Design review of the part built by this model. Coordinates are the model's own, in mm. Face numbers are marked on the shaded views. A direction names the side the tool comes from. Give positions to 0.01 mm unless a question says otherwise; leave off trailing zeros. Loops run counter-clockwise (first coordinate to the right, second up) from the corner with the lowest first, then second, coordinate; pieces in that order, holes last. Notation, with made-up numbers: (62, 44.25) - (110, 44.25) arc R17 cw to (110, 71.25) - close; hole circle Ø4 at (38.25, 65.25). An arc over 180 degrees is marked (long way). Write each question's results on one line, items separated by ' | '.
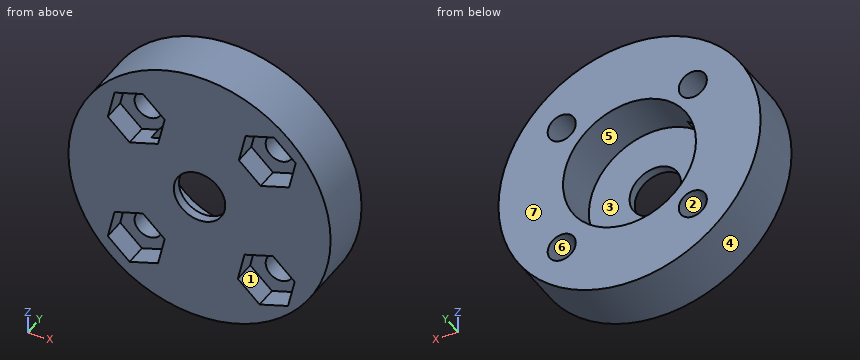
Autodesk Inventor part; units mm, degrees
ref_plane "YZ Plane" through (0, 0, 0) normal (1, 0, 0) x (0, 1, 0)
ref_plane "XZ Plane" through (0, 0, 0) normal (0, 1, 0) x (-1, 0, 0)
ref_plane "XY Plane" through (0, 0, 0) normal (0, 0, 1) x (1, 0, 0)
sketch "Эскиз1" plane through (0, 0, 0) normal (0, 1, 0) x (-1, 0, 0)
  circle A0 centre (0, 0) radius 14
  circle A1 centre (0, 0) radius 7.1
  circle A2 centre (6.7581, 6.7661) radius 1.5
  circle A3 centre (-7.2419, -7.2339) radius 1.5
  circle A4 centre (-7.2419, 6.7661) radius 1.5
  circle A5 centre (6.7581, -7.2339) radius 1.5
  circle A6 centre (0, 0) radius 2.75
  dimension "d0" = 28
  dimension "d1" = 14.2
  dimension "d4" = 5.5
extrude "Выдавливание2" add sketch "Эскиз1" along normal blind 6 contours A0
extrude "Выдавливание3" add sketch "Эскиз1" along normal blind 1 contours A1
sketch "Эскиз2" plane through (0, 0, 0) normal (0, -1, 0) x (1, 0, 0)
  line L0 (-9.0814, -5.0692) -> (-6.0451, -4.1396)
  line L1 (-6.0451, -4.1396) -> (-3.7219, -6.3042)
  line L2 (-3.7219, -6.3042) -> (-4.4349, -9.3986)
  line L3 (-4.4349, -9.3986) -> (-7.4712, -10.3282)
  line L4 (-7.4712, -10.3282) -> (-9.7944, -8.1636)
  line L5 (-9.7944, -8.1636) -> (-9.0814, -5.0692)
  circle A0 centre (-6.7581, -7.2339) radius 1.5
  circle A1 centre (-6.7581, 6.7661) radius 1.5
  circle A2 centre (7.2419, 6.7661) radius 1.5
  circle A3 centre (7.2419, -7.2339) radius 1.5
  line L6 (-9.0814, 8.9308) -> (-6.0451, 9.8604)
  line L7 (-6.0451, 9.8604) -> (-3.7219, 7.6958)
  line L8 (-3.7219, 7.6958) -> (-4.4349, 4.6014)
  line L9 (-4.4349, 4.6014) -> (-7.4712, 3.6718)
  line L10 (-7.4712, 3.6718) -> (-9.7944, 5.8364)
  line L11 (-9.7944, 5.8364) -> (-9.0814, 8.9308)
  line L12 (4.9186, 8.9308) -> (7.9549, 9.8604)
  line L13 (7.9549, 9.8604) -> (10.2781, 7.6958)
  line L14 (10.2781, 7.6958) -> (9.5651, 4.6014)
  line L15 (9.5651, 4.6014) -> (6.5288, 3.6718)
  line L16 (6.5288, 3.6718) -> (4.2056, 5.8364)
  line L17 (4.2056, 5.8364) -> (4.9186, 8.9308)
  line L18 (4.8052, -5.0148) -> (7.8414, -4.0851)
  line L19 (7.8414, -4.0851) -> (10.1647, -6.2498)
  line L20 (10.1647, -6.2498) -> (9.4517, -9.3441)
  line L21 (9.4517, -9.3441) -> (6.4154, -10.2738)
  line L22 (6.4154, -10.2738) -> (4.0921, -8.1091)
  line L23 (4.0921, -8.1091) -> (4.8052, -5.0148)
  line L24 (-9.0814, -5.0692) -> (-6.0451, -4.1396)
  line L25 (-6.0451, -4.1396) -> (-3.7219, -6.3042)
  line L26 (-3.7219, -6.3042) -> (-4.4349, -9.3986)
  line L27 (-4.4349, -9.3986) -> (-7.4712, -10.3282)
  line L28 (-7.4712, -10.3282) -> (-9.7944, -8.1636)
  line L29 (-9.7944, -8.1636) -> (-9.0814, -5.0692)
  point P0 (0, 0)
  dimension "d9" = 5.5
  dimension "d12" = 5.5
  dimension "d13" = 5.5
  dimension "d14" = 5.5
  dimension "d15" = 5.5
extrude "Выдавливание4" cut sketch "Эскиз2" against normal blind 2.4 contours L0 L1 L2 L3 L4 L5 | A1 | L6 L7 L8 L9 L10 L11 | L12 L13 L14 L15 L16 L17 | L18 L19 L20 L21 L22 L23
properties part number "rhtgt; gjlibgybrf"
(1) Wall thickness on line 1 along X through (y, z) = (1.8, 8); line 2 along Z through (x, y) = (8.5, 1.8); line 3 along Z through (x, y) = (0, 2.3): over which ranges is each line inside the solid? List them lowest first. Write a range as from..to.
Answers below:
line 1: -11.49..-9.3, -4.05..4.7, 9.95..11.49 | line 2: -11.12..-9.64, -4.7..4.28, 9.35..11.12 | line 3: -14..-7.1, 7.1..14
(2) Take a section at D-D on y = 4.85. Give the boundary of the cut face in (x, z), plus the area to 3 significant figures.
Answers below:
outline: circle Ø28 at (0, 0); hole circle Ø3 at (-6.76, -7.23); hole circle Ø3 at (-6.76, 6.77); hole circle Ø14.2 at (0, 0); hole circle Ø3 at (7.24, -7.23); hole circle Ø3 at (7.24, 6.77) | area: 429 mm2
(3) Draft analysis for pull direction Z (two halves, no side actions). For the marked faces 4, 5, 6 and 7, state which applies: pulls with the +Z half, pulls with the -Z half, needs draft (parallel to the pull), parting line crosses it, or undercut.
Answers below:
face 4: parting line crosses it | face 5: undercut | face 6: undercut | face 7: needs draft
(4) Tool access review of the marked faces 1, 2 and 3: name each direction out of +Z, -Z, +X, -X, +Y, -Y from which nothing blocks a thin tool from reaching the whole face with its end or side.
Answers below:
face 1: -Y | face 2: +Y, -Y | face 3: +Y
(5) Take a section at B-B on x = 0. Give the boundary of the cut face in (y, z), plus the area to 3 significant figures.
Answers below:
outline: (0, -14) - (6, -14) - (6, -7.1) - (1, -7.1) - (1, -2.75) - (0, -2.75) - close; (0, 2.75) - (1, 2.75) - (1, 7.1) - (6, 7.1) - (6, 14) - (0, 14) - close | area: 91.5 mm2
(6) Take a section at C-C on y = 2. Give the boundary of the cut face in (x, z), plus the area to 3 significant figures.
Answers below:
outline: circle Ø28 at (0, 0); hole (-9.79, -8.16) - (-7.47, -10.33) - (-4.43, -9.4) - (-3.72, -6.3) - (-6.05, -4.14) - (-9.08, -5.07) - close; hole (-9.79, 5.84) - (-7.47, 3.67) - (-5.72, 4.21) arc R7.1 ccw to (4.74, -5.28) - (4.09, -8.11) - (6.42, -10.27) - (9.45, -9.34) - (10.16, -6.25) - (7.84, -4.09) - (5.12, -4.92) arc R7.1 ccw to (-4.17, 5.75) - (-3.72, 7.7) - (-6.05, 9.86) - (-9.08, 8.93) - close; hole (4.21, 5.84) - (6.53, 3.67) - (9.57, 4.6) - (10.28, 7.7) - (7.95, 9.86) - (4.92, 8.93) - close | area: 353 mm2
(7) Insertion check: P1, Ø3.5, axis at x = 7.24, z = 6.77, coming from the -Y side; P2, Ø3, axis at y = 4, z = -6.5, coming from the +X side. Each pin has a flat end and moves straight along its axis. Give the tip position at first contact, or say it passes through.
Answers below:
P1: y = 2.4 | P2: x = 13.08
(8) Take a section at A-A on z = 0. Give the boundary of the cut face in (x, y).
Answers below:
outline: (-14, 0) - (-2.75, 0) - (-2.75, 1) - (-7.1, 1) - (-7.1, 6) - (-14, 6) - close; (2.75, 0) - (14, 0) - (14, 6) - (7.1, 6) - (7.1, 1) - (2.75, 1) - close
